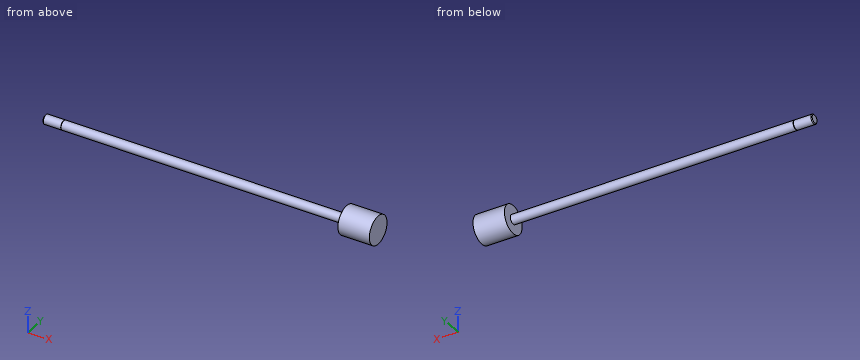
Autodesk Inventor part; units mm, degrees
ref_plane "rod_cp_XY" through (0, 0, 0) normal (1, 0, 0) x (0, 0, -1)
ref_plane "rod_cp_YZ" through (0, 0, 0) normal (0, 0, -1) x (0, 1, 0)
ref_plane "rod_cp_ZX" through (0, 0, 0) normal (0, 1, 0) x (1, 0, 0)
sketch "Sketch_1" plane through (0, 0, 0) normal (0, 0, 1) x (1, 0, 0)
  line L0 (214.3252, 0) -> (0, 0)
  line L1 (0, 0) -> (0, 3.175)
  line L2 (0, 3.175) -> (192.8876, 3.175)
  line L3 (192.8876, 3.175) -> (192.8876, 9.6203)
  line L4 (192.8876, 9.6203) -> (214.3252, 9.6203)
  line L5 (214.3252, 9.6203) -> (214.3252, 0)
  line L6 (214.3252, 0) -> (0, 0)
revolve "Revolution1" add sketch "Sketch_1" angle 360 about axis through (214.3252, 0, 0) along (1, 0, 0)
sketch "Sketch_3" plane through (0, 0, 0) normal (0, 0, 1) x (1, 0, 0)
  line L0 (0, 0) -> (-12.7, 0)
  line L1 (-12.7, 0) -> (-12.7, 2.634)
  line L2 (-12.7, 2.634) -> (-12.159, 3.175)
  line L3 (-12.159, 3.175) -> (0, 3.175)
  line L4 (0, 3.175) -> (0, 0)
  line L5 (0, 0) -> (-12.7, 0)
revolve "Revolution2" add sketch "Sketch_3" angle 360 about axis through (0, 0, 0) along (1, 0, 0)
thread "Thread1"
sketch "Sketch_30" plane through (0, 0, 0) normal (0, 0, 1) x (1, 0, 0)
  line L0 (0, 0) -> (-0.254, 0)
  line L1 (-0.254, 3.429) -> (-0.254, 2.921)
  line L2 (-0.254, 2.921) -> (0, 2.921)
  line L3 (0, 2.921) -> (0, 3.429)
  line L4 (0, 3.429) -> (-0.254, 3.429)
revolve "Revolution3" cut sketch "Sketch_30" angle 360 about axis through (0, 0, 0) along (1, 0, 0)
ref_plane "rod_cp_XY" through (0, 0, 0) normal (1, 0, 0) x (0, 0, -1)
ref_plane "rod_cp_YZ" through (0, 0, 0) normal (0, 0, -1) x (0, 1, 0)
ref_plane "rod_cp_ZX" through (0, 0, 0) normal (0, 1, 0) x (1, 0, 0)
ref_plane "to_rod_clevis_XY" through (-12.7, 0, 0) normal (1, 0, 0) x (0, 0, -1)
ref_plane "to_rod_clevis_YZ" through (-12.7, 0, 0) normal (0, 0, -1) x (0, 1, 0)
ref_plane "to_rod_clevis_ZX" through (-12.7, 0, 0) normal (0, 1, 0) x (1, 0, 0)
ref_plane "rl2_XY" through (0, 0, 0) normal (1, 0, 0) x (0, 0, -1)
ref_plane "rl2_YZ" through (0, 0, 0) normal (0, 0, -1) x (0, 1, 0)
ref_plane "rl2_ZX" through (0, 0, 0) normal (0, 1, 0) x (1, 0, 0)
ref_plane "rl1_XY" through (-12.7, 0, 0) normal (1, 0, 0) x (0, 0, -1)
ref_plane "rl1_YZ" through (-12.7, 0, 0) normal (0, 0, -1) x (0, 1, 0)
ref_plane "rl1_ZX" through (-12.7, 0, 0) normal (0, 1, 0) x (1, 0, 0)
ref_plane "thd1_XY" through (-12.7, 3.175, 0) normal (1, 0, 0) x (0, 0, -1)
ref_plane "thd1_YZ" through (-12.7, 3.175, 0) normal (0, 0, -1) x (0, 1, 0)
ref_plane "thd1_ZX" through (-12.7, 3.175, 0) normal (0, 1, 0) x (1, 0, 0)
ref_plane "thd2_XY" through (-12.7, -3.175, 0) normal (1, 0, 0) x (0, 0, -1)
ref_plane "thd2_YZ" through (-12.7, -3.175, 0) normal (0, 0, -1) x (0, 1, 0)
ref_plane "thd2_ZX" through (-12.7, -3.175, 0) normal (0, 1, 0) x (1, 0, 0)
ref_plane "dia1_XY" through (0, 3.175, 0) normal (1, 0, 0) x (0, 0, -1)
ref_plane "dia1_YZ" through (0, 3.175, 0) normal (0, 0, -1) x (0, 1, 0)
ref_plane "dia1_ZX" through (0, 3.175, 0) normal (0, 1, 0) x (1, 0, 0)
ref_plane "dia2_XY" through (0, -3.175, 0) normal (1, 0, 0) x (0, 0, -1)
ref_plane "dia2_YZ" through (0, -3.175, 0) normal (0, 0, -1) x (0, 1, 0)
ref_plane "dia2_ZX" through (0, -3.175, 0) normal (0, 1, 0) x (1, 0, 0)
ref_plane "hh1_XY" through (244.4496, 0, 0) normal (0, 0, 1) x (1, 0, 0)
ref_plane "hh1_YZ" through (244.4496, 0, 0) normal (1, 0, 0) x (0, 1, 0)
ref_plane "hh1_ZX" through (244.4496, 0, 0) normal (0, 1, 0) x (0, 0, 1)
ref_plane "hh2_XY" through (250.8504, 0, 0) normal (0, 0, 1) x (1, 0, 0)
ref_plane "hh2_YZ" through (250.8504, 0, 0) normal (1, 0, 0) x (0, 1, 0)
ref_plane "hh2_ZX" through (250.8504, 0, 0) normal (0, 1, 0) x (0, 0, 1)
ref_plane "dia12_XY" through (0, 0, 10.9537) normal (1, 0, 0) x (0, 0, -1)
ref_plane "dia12_YZ" through (0, 0, 10.9537) normal (0, 0, -1) x (0, 1, 0)
ref_plane "dia12_ZX" through (0, 0, 10.9537) normal (0, 1, 0) x (1, 0, 0)
ref_plane "dia22_XY" through (0, 0, -10.9537) normal (1, 0, 0) x (0, 0, -1)
ref_plane "dia22_YZ" through (0, 0, -10.9537) normal (0, 0, -1) x (0, 1, 0)
ref_plane "dia22_ZX" through (0, 0, -10.9537) normal (0, 1, 0) x (1, 0, 0)
properties part number "046-DXP0_rod"
The listing builds one solid part. Answer for the finished solid, in the listing's coordinates (mm). Coordinates: 2 decimals unless noted, no trailing zeros. Order: outer loops, then holes, each group sorted by start corner. A loop starts at its lowest first (then second) coordinate and runs counter-clockwise, first axis right, second up. Notation, with made-up numbers: M 35,-12 L 73,-12 A19 ccw 73,18 Z; hole C 21.5,36.5 d2. An arc over 180 degrees is marked long. Answer as a JSON object with one key per item and string values. Group by question number.
1. Flat-ended cylindrical pins translate along their axes: P1, Ø4, axis at x = 33, y = 4.5, coming from the +Z side; P2, Ø10, axis at x = 48, z = 6.5, coming from the -Y side; P3, Ø8, axis at x = 55, z = -3, coming from the +Y side (3 decimals). Find the tip coordinate at first contact, or state that the pin passes through.
2. Section C-C on x = 98.5 is taken. Write down the section's boundary in (y, z) (3 decimals), then the cut area to 3 significant figures.
3. Straight lines are drawn through the part: line 1 (X direction, y = 1.5, z = 6.25); line 2 (Z direction, x = 161, y = -2.75); line 3 (Z direction, x = 197.5, y = -5). For each, find the intervals that lie inside material, in ascending order.
4. Section A-A on y = 0 is taken. Write down the section's boundary in (x, z) (3 decimals).
Values follow:
{
 "1": {"P1": "z = 1.96", "P2": "y = -2.8", "P3": "y = 3.175"},
 "2": {"outline": "C 0,0 d6.35", "area": "31.7 mm2"},
 "3": {"line 1": "192.89 to 214.33", "line 2": "-1.59 to 1.59", "line 3": "-8.22 to 8.22"},
 "4": {"outline": "M -12.7,-2.634 L -12.159,-3.175 L -0.254,-3.175 L -0.254,-2.921 L 0,-2.921 L 0,-3.175 L 192.888,-3.175 L 192.888,-9.62 L 214.325,-9.62 L 214.325,9.62 L 192.888,9.62 L 192.888,3.175 L 0,3.175 L 0,2.921 L -0.254,2.921 L -0.254,3.175 L -12.159,3.175 L -12.7,2.634 Z"}
}
